from build123d import *

# Parameters (mm, degrees)
SKETCH1_W           = 15.85
SKETCH1_H           = 7.75
BOSS_EXTRUDE1_DEPTH = 9.6
SKETCH2_R           = 2.45
BOSS_EXTRUDE2_DEPTH = 1.8
SHELL1_T            = -1.5
SKETCH3_R           = 1.5
BOSS_EXTRUDE3_DEPTH = 7.9


with BuildPart() as part:
    # Sketch1 → Boss-Extrude1 (new body)
    with BuildSketch(Plane(origin=(0, 0, 0), x_dir=(1, 0, 0), z_dir=(0, 1, 0))):
        Rectangle(SKETCH1_W, SKETCH1_H)
    extrude(amount=-BOSS_EXTRUDE1_DEPTH)

    # Sketch2 → Boss-Extrude2 (add)
    with BuildSketch(Plane(origin=(0, 0, 0), x_dir=(1, 0, 0), z_dir=(0, 1, 0))):
        with Locations(Location((-3.9625, 0, 0), (0, 0, 270))):
            Circle(SKETCH2_R)
        with Locations(Location((3.9625, 0, 0), (0, 0, 270))):
            Circle(SKETCH2_R)
    extrude(amount=BOSS_EXTRUDE2_DEPTH)

    # Shell1
    shell1_openings = [part.faces().sort_by_distance(p)[0] for p in [
        (0, -9.6, 0),
    ]]
    offset(amount=SHELL1_T, openings=shell1_openings, kind=Kind.INTERSECTION)

    # Sketch3 → Boss-Extrude3 (add)
    with BuildSketch(Plane.XZ.offset(1.5)):
        with Locations(Location((0, 0, 0), (0, 0, 90))):
            Circle(SKETCH3_R)
    extrude(amount=BOSS_EXTRUDE3_DEPTH)


solid = part.part
For this review, take the finished solid that the model builds, in its own axes (mm). A direction names the side the tool comes from. Give positions to 0.01 mm unless a question says otherwise; leave off trailing zeros. Loops run counter-clockwise (first coordinate to the right, second up) from the corner with the lowest first, then second, coordinate; pieces in that order, holes last.
Item 1: Draft analysis for pull direction X (two halves, no side actions). For faces 4 (the flat face through (7.925, -5, 0)), 5 (the flat face through (-4, 1.8, 0)), 6 (the cylindrical face through (1.57, 0.89, -0.53)), state which applies: +X half, -X half, draft (parallel to the pull), parting line (faces both ways), or undercut.
Item 2: Take a section at D-D, the plane y = 1. State the section outline as (x, z) points.
Item 3: Take a section at A-A, the plane y = -2.25. State the section outline as (x, z) points (3 decimals), and give its area (3 significant figures).
Item 4: Take a section at C-C, the plane x = 0. State the section outline as (y, z) points (3 decimals).
Item 5: Insertion check: pin 1 (0.6 mm diameter, centred on x = 4, z = 0, fed in from -Y); pin 2 (2.5 mm diameter, centred on x = -3.96, z = 0, fed in from -Y); pin 3 (0.9 mm diameter, centred on x = -0.5, z = -0.5, fed in from -Y). Each pin has a flat end and moves straight along its axis. Give the tip position at first contact, or say it passes through.
Item 6: For line 1 along X through (y, z) = (-1.1, 0) (1 decimal); line 2 along X through (y, z) = (-9, 2.25) (3 decimals); line 3 along Z through (x, y) = (0.75, -3.75) (3 decimals), list the stretches that pass through material, from the lowest coordinate up.
Item 7: Tool access review of faces 1 (the flat face through (0, -9.6, -3)), 2 (the flat face through (0, 0, 0)), 3 (the flat face through (0, -9.4, 0)): name each direction out of +Z, -Z, +X, -X, +Y, -Y from which nothing blocks a thin tool from reaching the whole face with its end or side.
Item 8: Take a section at B-B, the plane z = 0. State the section outline as (x, y) points (1 decimal), and give its area (3 significant figures).
Calculated:
1. face 4: +X half
1. face 5: draft
1. face 6: undercut
2. outline: circle Ø4.9 at (-3.96, 0); circle Ø4.9 at (3.96, 0)
3. outline: (-7.925, -3.875) - (7.925, -3.875) - (7.925, 3.875) - (-7.925, 3.875) - close; circle Ø3 at (0, 0); hole (-6.425, -2.375) - (6.425, -2.375) - (6.425, 2.375) - (-6.425, 2.375) - close
3. area: 68.9 mm2
4. outline: (-9.6, -3.875) - (0, -3.875) - (0, 3.875) - (-9.6, 3.875) - (-9.6, 2.375) - (-1.5, 2.375) - (-1.5, 1.5) - (-9.4, 1.5) - (-9.4, -1.5) - (-1.5, -1.5) - (-1.5, -2.375) - (-9.6, -2.375) - close
5. pin 1: stops at y = 0.3
5. pin 2: stops at y = -1.5
5. pin 3: stops at y = -9.4
6. line 1: x = -7.9 to -4.9, -3 to 3, 4.9 to 7.9
6. line 2: x = -7.925 to -6.425, 6.425 to 7.925
6. line 3: z = -3.875 to -2.375, -1.299 to 1.299, 2.375 to 3.875
7. face 1: +Z, -Z, +X, -X, -Y
7. face 2: +Y
7. face 3: -Y
8. outline: (-7.9, -9.6) - (-6.4, -9.6) - (-6.4, -1.5) - (-4.9, -1.5) - (-4.9, 0.3) - (-3, 0.3) - (-3, -1.5) - (-1.5, -1.5) - (-1.5, -9.4) - (1.5, -9.4) - (1.5, -1.5) - (3, -1.5) - (3, 0.3) - (4.9, 0.3) - (4.9, -1.5) - (6.4, -1.5) - (6.4, -9.6) - (7.9, -9.6) - (7.9, 0) - (6.4, 0) - (6.4, 1.8) - (1.5, 1.8) - (1.5, 0) - (-1.5, 0) - (-1.5, 1.8) - (-6.4, 1.8) - (-6.4, 0) - (-7.9, 0) - close
8. area: 82.6 mm2
